from build123d import *

# Parameters (mm, degrees)
BOSS_EXTRUDE1_DEPTH = 1.5875
FILLET1_R           = 3.175


with BuildPart() as part:
    # Sketch1 → Boss-Extrude1 (new body, symmetric)
    with BuildSketch(Plane(origin=(0, 0, 0), x_dir=(1, 0, 0), z_dir=(0, 1, 0))):
        with BuildLine():
            Line((6.35, 31.75), (6.35, -31.75))
            ThreePointArc((6.35, -31.75), (7.149186899, -41.406385517), (9.525, -50.8))
            Line((9.525, -50.8), (9.525, -82.55))
            Line((9.525, -82.55), (-9.525, -82.55))
            Line((-9.525, -82.55), (-9.525, -50.8))
            ThreePointArc((-9.525, -50.8), (-7.149186899, -41.406385517), (-6.35, -31.75))
            Line((-6.35, -31.75), (-6.35, 31.75))
            ThreePointArc((-6.35, 31.75), (-7.149186899, 41.406385517), (-9.525, 50.8))
            Line((-9.525, 50.8), (-9.525, 82.55))
            Line((-9.525, 82.55), (9.525, 82.55))
            Line((9.525, 82.55), (9.525, 50.8))
            ThreePointArc((9.525, 50.8), (7.149186899, 41.406385517), (6.35, 31.75))
        make_face()
    extrude(amount=BOSS_EXTRUDE1_DEPTH, both=True)

    # Fillet1
    fillet1_edges = [part.edges().sort_by_distance(p)[0] for p in [
        (9.525, 0, 82.55),
        (-9.525, 0, 82.55),
        (-9.525, 0, -82.55),
        (9.525, 0, -82.55),
    ]]
    fillet(fillet1_edges, radius=FILLET1_R)


solid = part.part
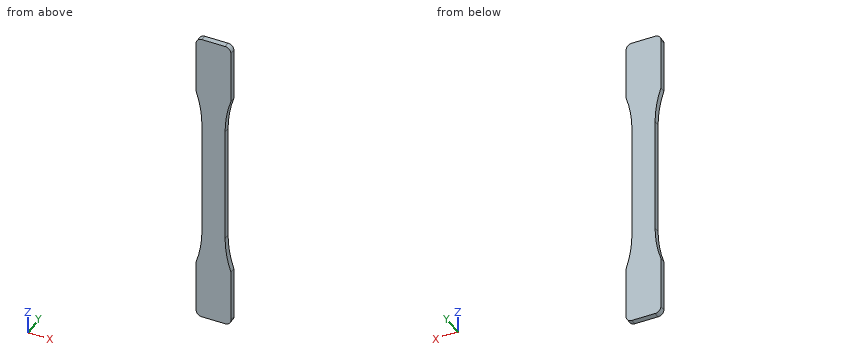
Work out the finished part from the listing and answer in its coordinate system (mm). Give positions to 0.01 mm unless a question says otherwise; leave off trailing zeros. Loops run counter-clockwise (first coordinate to the right, second up) from the corner with the lowest first, then second, coordinate; pieces in that order, holes last. Notation, with made-up numbers: (46.5, -40) - (89.5, -40) arc R20 ccw to (89.5, -8) - close; hole circle Ø1 at (22, 30). An arc over 180 degrees is marked (long way). Answer in a Markdown table with one row per item. Add a question column.
Q1. Consider line 1 along X through (y, z) = (0.65, 31.5). Determine where the line is inside the solid, lowest interval first.
Q2. This flat-tipped pin is pushed along its axis until it touches: P1, Ø1, axis at y = 0.5, z = 38.5, coming from the -X side. Where does it stop, or does it pass through?
Q3. The part is cut by section A-A (x = -7.75). Determine the outline of the cut face in (y, z), and give its area (3 significant figures).
Q4. The part is cut by section D-D (z = 43). Determine the outline of the cut face in (x, y).
Q5. The part is cut by section C-C (z = -6). Determine the outline of the cut face in (x, y).
Solution:
| question | item | result |
|---|---|---|
| 1 | line 1 | x = -6.35 to 6.35 |
| 2 | P1 | stops at x = -6.8 |
| 3 | outline | (-1.59, -82.22) - (1.59, -82.22) - (1.59, -44.5) - (-1.59, -44.5) - close; (-1.59, 44.5) - (1.59, 44.5) - (1.59, 82.22) - (-1.59, 82.22) - close |
| 3 | area | 240 mm² |
| 4 | outline | (-7.44, -1.59) - (7.44, -1.59) - (7.44, 1.59) - (-7.44, 1.59) - close |
| 5 | outline | (-6.35, -1.59) - (6.35, -1.59) - (6.35, 1.59) - (-6.35, 1.59) - close |
